Verification items for this drawing (mm, ordinates from the low corner). A direction names the side the tool comes from. Round coordinates to 2 decimals unless told otherwise and drop trailing zeros. Loops run counter-clockwise (first coordinate to the right, second up) from the corner with the lowest first, then second, coordinate; pieces in that order, holes last. Notation, with made-up numbers: (44, -18.5) -> (60, -18.5) arc R5 cw to (60, -9.5) -> close; hole circle Ø3 at (49.25, 16.5). An arc over 180 degrees is marked (long way). Use a Markdown table: item, result. Add a question column.
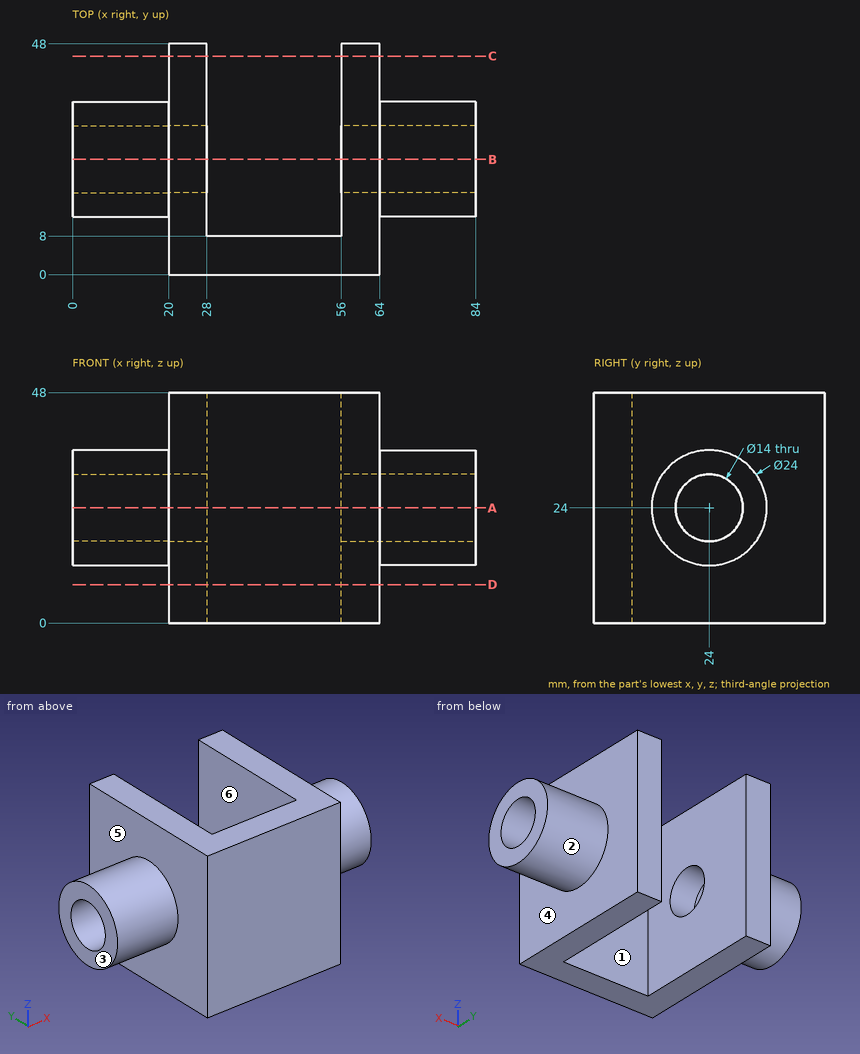
1) Sectioned sample at A-A on z = 24. Enter the section's corners in (x, y), then the cut area to 3 significant figures.
2) Sectioned sample at B-B on y = 24. Enter the section's corners in (x, z), then the cut area to 3 significant figures.
3) Release check for a two-part mould opening along X. For the marked faces 1, 2 and 3 record: released by +X, released by -X, zero draft, split by the parting line, or undercut.
4) Sectioned sample at D-D on z = 8. Enter the section's corners in (x, y), then the cut area to 3 significant figures.
5) Thickness scan on line 1 (Z direction, x = 13, y = 24); line 2 (Y direction, x = 62, z = 24); line 3 (X direction, y = 13, z = 9). Record the ranges inside material, lowest first.
6) Sectioned sample at C-C on y = 45.5. Enter the section's corners in (x, z).
7) Access from +Z, -Z, +X, -X, +Y, -Y to the whole of each face (thin tool, end or side, straight path). Record for the marked faces 4, 5 and 6.
8) Go/stop test with flat-tipped pins: pin 1 (1.5 mm diameter, centred on x = 67.5, y = 31.5, fed in from +Z); pin 2 (1 mm diameter, centred on x = 38, z = 20.5, fed in from +Y); pin 3 (4 mm diameter, centred on y = 23, z = 39, fed in from +X). Record where each tip stops, or that it passes through.
Geometry results:
| question | item | result |
|---|---|---|
| 1 | outline | (0, 12) -> (20, 12) -> (20, 0) -> (64, 0) -> (64, 12) -> (84, 12) -> (84, 17) -> (56, 17) -> (56, 8) -> (28, 8) -> (28, 17) -> (0, 17) -> close; (0, 31) -> (28, 31) -> (28, 48) -> (20, 48) -> (20, 36) -> (0, 36) -> close; (56, 31) -> (84, 31) -> (84, 36) -> (64, 36) -> (64, 48) -> (56, 48) -> close |
| 1 | area | 1,170 mm^2 |
| 2 | outline | (0, 12) -> (20, 12) -> (20, 0) -> (28, 0) -> (28, 17) -> (0, 17) -> close; (0, 31) -> (28, 31) -> (28, 48) -> (20, 48) -> (20, 36) -> (0, 36) -> close; (56, 0) -> (64, 0) -> (64, 12) -> (84, 12) -> (84, 17) -> (56, 17) -> close; (56, 31) -> (84, 31) -> (84, 36) -> (64, 36) -> (64, 48) -> (56, 48) -> close |
| 2 | area | 944 mm^2 |
| 3 | face 1 | undercut |
| 3 | face 2 | zero draft |
| 3 | face 3 | released by -X |
| 4 | outline | (20, 0) -> (64, 0) -> (64, 48) -> (56, 48) -> (56, 8) -> (28, 8) -> (28, 48) -> (20, 48) -> close |
| 4 | area | 992 mm^2 |
| 5 | line 1 | 12 to 17, 31 to 36 |
| 5 | line 2 | 0 to 17, 31 to 48 |
| 5 | line 3 | 20 to 28, 56 to 64 |
| 6 | outline | (20, 0) -> (28, 0) -> (28, 48) -> (20, 48) -> close; (56, 0) -> (64, 0) -> (64, 48) -> (56, 48) -> close |
| 7 | face 4 | +X |
| 7 | face 5 | -X |
| 7 | face 6 | +Z, -Z, +Y |
| 8 | pin 1 | z = 33.92 |
| 8 | pin 2 | y = 8 |
| 8 | pin 3 | x = 64 |
